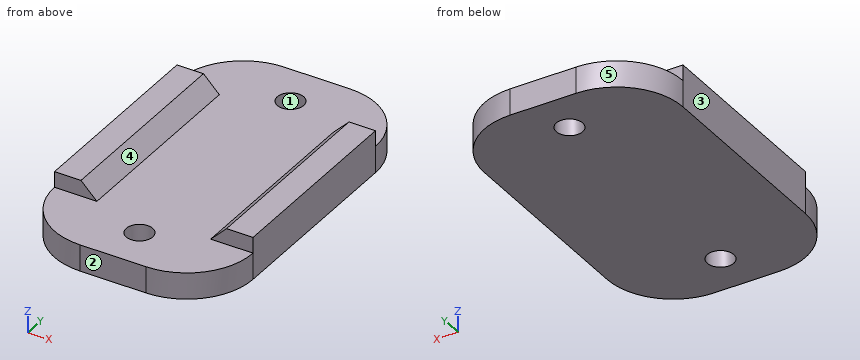
Autodesk Inventor part; units mm, degrees
ref_plane "YZ Plane" through (0, 0, 0) normal (1, 0, 0) x (0, 1, 0)
ref_plane "XZ Plane" through (0, 0, 0) normal (0, 1, 0) x (-1, 0, 0)
ref_plane "XY Plane" through (0, 0, 0) normal (0, 0, 1) x (1, 0, 0)
sketch "Эскиз1" plane through (0, 0, 0) normal (0, 0, 1) x (1, 0, 0)
  circle A0 centre (0, 0) radius 6
  line L0 (-7.5, 12.5) -> (7.5, 12.5)
  line L1 (7.5, 12.5) -> (7.5, -12.5)
  line L2 (7.5, -12.5) -> (-7.5, -12.5)
  line L3 (-7.5, -12.5) -> (-7.5, 12.5)
  line L4 (-7.5, 12.5) -> (7.5, -12.5) construction
  line L5 (7.5, 12.5) -> (-7.5, -12.5) construction
  line L6 (0, 6) -> (0, 12.5)
  line L7 (0, -6) -> (0, -12.5)
  circle A1 centre (0, 9.25) radius 1
  circle A2 centre (0, -9.25) radius 1
  dimension "d0" = 12
  dimension "d1" = 15
  dimension "d2" = 25
  dimension "d31" = 2
  dimension "d32" = 2
extrude "Выдавливание1" add sketch "Эскиз1" along normal blind 2 contours A0 | A0 L6 A1 L0 L1 L2 L7 A2 | A0 L7 A2 L2 L3 L0 L6 A1
fillet "Сопряжение6" radius 5 4 edges at (-7.5, -12.5, 1) (-7.5, 12.5, 1) (7.5, 12.5, 1) (7.5, -12.5, 1)
sketch "Эскиз7" plane through (0, 0, 2) normal (0, 0, 1) x (1, 0, 0)
  circle A0 centre (0, 0) radius 4
  circle A1 centre (0, 0) radius 6
  line L0 (-7.5, 7.5) -> (-7.5, -7.5)
  line L1 (-7.5, 7.5) -> (-5.5, 7.5)
  line L2 (-5.5, 7.5) -> (-5.5, -7.5)
  line L3 (-5.5, -7.5) -> (-7.5, -7.5)
  line L4 (-7.5, -7.5) -> (-7.5, 7.5)
  arc A2 (7.5, 7.5) -> (2.5, 12.5) centre (2.5, 7.5) ccw
  line L5 (7.5, 7.5) -> (5.5, 7.5)
  line L6 (5.5, 7.5) -> (5.5, -7.5)
  line L7 (5.5, -7.5) -> (7.5, -7.5)
  line L8 (7.5, -7.5) -> (7.5, 7.5)
  dimension "d34" = 8
  dimension "d35" = 12
  dimension "d36" = 2
  dimension "d37" = 2
extrude "Выдавливание7" add sketch "Эскиз7" along normal blind 1.2 contours A1 L6 | A1 L6 L5 L8 L7 | L2 A1 | A1 L2 L3 L0 L1
chamfer "Фаска1" distance 1.2 angle 45 2 edges at (5.5, 0, 2) (-5.5, 0, 2)
properties part number "led_cap"
Part model, mm, in its own coordinate system. Face numbers are marked on the shaded views. A direction names the side the tool comes from. Give positions to 0.01 mm unless a question says otherwise; leave off trailing zeros. Write each loop counter-clockwise with the first axis right and the second up, starting at its lowest first coordinate (ties: lowest second). Pieces come first, ordered by that corner, then holes. Notation, with made-up numbers: M 13.5,13 L 67.5,13 A18 ccw 67.5,48 Z; hole C 41.5,50.25 d10. An arc over 180 degrees is marked long. Use CSV: the item, a comma, the result in double quotes.
Item 1: Slice it at D-D on z = 2.95. Write the cut outline in (x, y).
Taken from the geometry:
outline,"M -7.5,-7.5 L -5.25,-7.5 L -5.25,7.5 L -7.5,7.5 Z; M 5.25,-7.5 L 7.5,-7.5 L 7.5,7.5 L 5.25,7.5 Z"
Item 2: Slice it at B-B on y = 9.25. Write the cut outline in (x, z).
Taken from the geometry:
outline,"M -7.18,0 L -1,0 L -1,2 L -7.18,2 Z; M 1,0 L 7.18,0 L 7.18,2 L 1,2 Z"
Item 3: Pull direction X, two halves, no side cores. Call the marked faces 1, 2 and 3: +X half, -X half, draft (parallel to the pull), parting line (faces both ways), or undercut.
Taken from the geometry:
face 1,"undercut"
face 2,"draft"
face 3,"-X half"
Item 4: Slice it at A-A on x = 0. Write the cut outline in (y, z).
Taken from the geometry:
outline,"M -12.5,0 L -10.25,0 L -10.25,2 L -12.5,2 Z; M -8.25,0 L 8.25,0 L 8.25,2 L -8.25,2 Z; M 10.25,0 L 12.5,0 L 12.5,2 L 10.25,2 Z"
Item 5: Pin check, flat tips, straight feed: P1, Ø1, axis at x = 3.5, z = 1, coming from the +Y side; P2, Ø1.3, axis at x = 5, z = 2.5, coming from the -Y side; P3, Ø0.6, axis at x = -5.5, z = 3, coming from the -Y side. Stop position of each tip, or through.
Taken from the geometry:
P1,"stops at y = 12.47"
P2,"stops at y = -12.04"
P3,"stops at y = -7.5"
Item 6: Drill centre lines: probe 1 along Y at (x, z) = (0, 0.6); probe 2 along Y at (x, z) = (5.5, 2.8); probe 3 along Z at (x, y) = (-1, -1.5). Where is each one in solid material? Low to high.
Taken from the geometry:
probe 1,"y = -12.5 to -10.25, -8.25 to 8.25, 10.25 to 12.5"
probe 2,"y = -7.5 to 7.5"
probe 3,"z = 0 to 2"
Item 7: Slice it at C-C on z = 1.1. Write the cut outline in (x, y), plus the area to 3 significant figures.
Taken from the geometry:
outline,"M -7.5,-7.5 A5 ccw -2.5,-12.5 L 2.5,-12.5 A5 ccw 7.5,-7.5 L 7.5,7.5 A5 ccw 2.5,12.5 L -2.5,12.5 A5 ccw -7.5,7.5 Z; hole C 0,-9.25 d2; hole C 0,9.25 d2"
area,"347 mm²"
Item 8: Which spindle directions (+Z, -Z, +X, -X, +Y, -Y) get a long thin tool onto all of the face, cutting with end or side? Do the marked faces 4 and 5. Say none if no direction does.
Taken from the geometry:
face 4,"+Z, +Y, -Y"
face 5,"+Z, -Z, -X, +Y"
